```python
from build123d import *

# Parameters (mm, degrees)
SKETCH1_W               = 72.154028999
SKETCH1_H               = 39.439030188
BOSS_EXTRUDE1_DEPTH     = 2.5
CUT_EXTRUDE1_DEPTH      = 83.26719275
CUT_EXTRUDE1_DEPTH_BACK = 15
SKETCH2_W               = 72.154028999
SKETCH2_H               = 39.439030188
CHAMFER1_SIZE           = 0.5
CHAMFER2_SIZE           = 0.5
CUT_EXTRUDE2_DEPTH      = 10


with BuildPart() as part:
    # Sketch1 → Boss-Extrude1 (new body)
    with BuildSketch(Plane(origin=(0, 0, 0), x_dir=(1, 0, 0), z_dir=(0, 1, 0))):
        with Locations((36.0770145, 19.719515094)):
            Rectangle(SKETCH1_W, SKETCH1_H)
    extrude(amount=BOSS_EXTRUDE1_DEPTH)

    # Sketch2 → Cut-Extrude1 (cut, two sides: drawn at the far end of the back side and taken through both)
    with BuildSketch(Plane(origin=(0, 2.5, 0), x_dir=(1, 0, 0), z_dir=(0, 1, 0)).offset(-CUT_EXTRUDE1_DEPTH_BACK)):
        with Locations((36.0770145, 19.719515094)):
            Rectangle(SKETCH2_W, SKETCH2_H)
        with BuildLine():
            Line((38.3020145, 17.735642877), (38.3020145, 19.460642877))
            ThreePointArc((38.3020145, 19.460642877), (36.0770145, 21.685642877), (33.8520145, 19.460642877))
            Line((33.8520145, 19.460642877), (33.8520145, 17.735642877))
            Line((33.8520145, 17.735642877), (29.362179375, 17.735642877))
            Line((29.362179375, 17.735642877), (29.362179375, 19.735642877))
            Line((29.362179375, 19.735642877), (32.362179375, 19.735642877))
            Line((32.362179375, 19.735642877), (32.362179375, 23.185642877))
            Line((32.362179375, 23.185642877), (39.791849624, 23.185642877))
            Line((39.791849624, 23.185642877), (39.791849624, 19.735642877))
            Line((39.791849624, 19.735642877), (42.791849624, 19.735642877))
            Line((42.791849624, 19.735642877), (42.791849624, 17.735642877))
            Line((42.791849624, 17.735642877), (38.3020145, 17.735642877))
        make_face(mode=Mode.SUBTRACT)
    extrude(amount=CUT_EXTRUDE1_DEPTH + CUT_EXTRUDE1_DEPTH_BACK, mode=Mode.SUBTRACT)

    # Chamfer1
    chamfer1_edges = [part.edges().sort_by_distance(p)[0] for p in [
        (36.0770145, 0, -21.685642877),
        (33.8520145, 0, -18.598142877),
        (38.3020145, 0, -18.598142877),
    ]]
    chamfer(chamfer1_edges, length=CHAMFER1_SIZE)

    # Chamfer2
    chamfer2_edges = [part.edges().sort_by_distance(p)[0] for p in [
        (38.3020145, 2.5, -18.598142877),
        (33.8520145, 2.5, -18.598142877),
        (36.0770145, 2.5, -21.685642877),
    ]]
    chamfer(chamfer2_edges, length=CHAMFER2_SIZE)

    # Sketch4 → Cut-Extrude2 (cut)
    with BuildSketch(Plane(origin=(0, 0, -19.735642877), x_dir=(-1, 0, 0), z_dir=(0, 0, -1))):
        with BuildLine():
            ThreePointArc((-42.341849624, 1.25), (-41.291849624, 0.2), (-40.241849624, 1.25))
            Line((-40.241849624, 1.25), (-42.341849624, 1.25))
        make_face()
        with BuildLine():
            Line((-42.341849624, 1.25), (-40.241849624, 1.25))
            ThreePointArc((-40.241849624, 1.25), (-41.291849624, 2.3), (-42.341849624, 1.25))
        make_face()
        with BuildLine():
            ThreePointArc((-29.812179375, 1.25), (-30.862179375, 2.3), (-31.912179375, 1.25))
            Line((-31.912179375, 1.25), (-29.812179375, 1.25))
        make_face()
        with BuildLine():
            Line((-29.812179375, 1.25), (-31.912179375, 1.25))
            ThreePointArc((-31.912179375, 1.25), (-30.862179375, 0.2), (-29.812179375, 1.25))
        make_face()
    extrude(amount=-CUT_EXTRUDE2_DEPTH, mode=Mode.SUBTRACT)


solid = part.part
```
The model under review builds one solid part; all positions refer to its coordinate system, in mm. A direction names the side the tool comes from. Round coordinates to 2 decimals unless told otherwise and drop trailing zeros. Write each loop counter-clockwise with the first axis right and the second up, starting at its lowest first coordinate (ties: lowest second). Pieces come first, ordered by that corner, then holes. Notation, with made-up numbers: (8.25, 22.5) -> (56.25, 22.5) arc R32 ccw to (56.25, 55.5) -> close; hole circle Ø9 at (-29, -14). An arc over 180 degrees is marked (long way). Use CSV: the item, a comma, the result in double quotes.
Q1. Mouldability with a two-part tool opening along X and no side actions: class faces 1 (the flat face through (42.792, 1, -19)), 2 (the flat face through (32.1, 1.2, -17.736)), 3 (the conical face through (36.025, 0.365, -21.82)) as released by +X, released by -X, zero draft, split by the parting line, or undercut.
Checks:
face 1,"released by +X"
face 2,"zero draft"
face 3,"undercut"
Q2. Consider section D-D (y = 1.85). State how many separate pieces and enclosed holes the cut face has, then the cut area to 3 significant figures.
Checks:
separate pieces,"3"
enclosed holes,"0"
area,"30.1 mm²"
Q3. For pin 1 Ø1.2 at (x, y) = (30.5, 2) entering from -Z; pin 2 Ø3 at (x, z) = (36.5, -19.5) entering from -Y, all flat-tipped, find the tip position at first contact; note any pin that passes through.
Checks:
pin 1,"z = -19.74"
pin 2,"through"
Q4. To check wall thickness, follow probe 1 along X at (y, z) = (2.05, -19.2); probe 2 along Z at (x, y) = (40.25, 0.15); probe 3 along Y at (x, z) = (40.5, -18.6). State the ranges of each line that lie inside material, in increasing order. Write a range as [from, to].
Checks:
probe 1,"[29.36, 30.18], [31.54, 33.8], [38.35, 40.61], [41.97, 42.79]"
probe 2,"[-19.74, -17.74]"
probe 3,"[0, 0.56], [1.94, 2.5]"
Q5. Consider section C-C (x = 30.75). Give the boundary of the cut face in (y, z).
Checks:
outline,"(0, -19.74) -> (0.21, -19.74) -> (0.21, -17.74) -> (0, -17.74) -> close; (2.29, -19.74) -> (2.5, -19.74) -> (2.5, -17.74) -> (2.29, -17.74) -> close"
Q6. For faces 4 (the flat face through (33.852, 1, -19)), 5 (the flat face through (39.792, 1, -21)), 6 (the flat face through (32.362, 1, -21)), list the 3-axis set-ups (+Z, -Z, +X, -X, +Y, -Y) from which the entire face can be reached by the end or side of a thin tool; tool diameter is ignored.
Checks:
face 4,"+Z, +Y, -Y"
face 5,"-Z, +X, +Y, -Y"
face 6,"-Z, -X, +Y, -Y"
Q7. Consider section B-B (y = 1.25). Give the boundary of the cut face in (x, z) (3 decimals), then the cut area to 3 significant figures.
Checks:
outline,"(29.362, -19.736) -> (29.812, -19.736) -> (29.812, -17.736) -> (29.362, -17.736) -> close; (31.912, -19.736) -> (32.362, -19.736) -> (32.362, -23.186) -> (39.792, -23.186) -> (39.792, -19.736) -> (40.242, -19.736) -> (40.242, -17.736) -> (38.302, -17.736) -> (38.302, -19.461) arc R2.225 cw to (33.852, -19.461) -> (33.852, -17.736) -> (31.912, -17.736) -> close; (42.342, -19.736) -> (42.792, -19.736) -> (42.792, -17.736) -> (42.342, -17.736) -> close"
area,"28.6 mm²"
Q8. Consider section A-A (z = -18.15). Give the boundary of the cut face in (x, y), then the cut area to 3 significant figures.
Checks:
outline,"(29.36, 0) -> (33.35, 0) -> (33.85, 0.5) -> (33.85, 2) -> (33.35, 2.5) -> (29.36, 2.5) -> close; (38.3, 0.5) -> (38.8, 0) -> (42.79, 0) -> (42.79, 2.5) -> (38.8, 2.5) -> (38.3, 2) -> close; hole circle Ø2.1 at (30.86, 1.25); hole circle Ø2.1 at (41.29, 1.25)"
area,"15.0 mm²"
